Geometry: final body of the model. Coordinates: model frame, mm. Face numbers are marked on the shaded views. A direction names the side the tool comes from. Round coordinates to 2 decimals unless told otherwise and drop trailing zeros. Order: outer loops, then holes, each group sorted by start corner. A loop starts at its lowest first (then second) coordinate and runs counter-clockwise, first axis right, second up. Notation, with made-up numbers: (9.5, -6.75) - (29.5, -6.75) arc R9 ccw to (29.5, 7.25) - close; hole circle Ø1 at (-16.75, 37.25). An arc over 180 degrees is marked (long way). Put each result on its own line as item: value. Start each with the question number.
(1) Access query for the marked faces 1 and 2. Directions: +Z, -Z, +X, -X, +Y, -Y. A direction counts if a zero-diameter tool reaches every point of the face in a straight line with its end or side. Return the directions, or none.
(2) Pin query (flat end, axial travel): P1, Ø6, axis at x = 8, z = 40, coming from the +Y side; P2, Ø5, axis at y = 11.75, z = 9.5, coming from the -X side; P3, Ø10.5, axis at x = 45, y = 5.5, coming from the -Z side. Return the tip coordinate at first contact, or that it passes through.
(3) Material intervals for L1, parallel to Y at x = 51.85, z = 40.5; L2, parallel to Z at x = 51, y = 11; L3, parallel to Z at x = 54.05, y = 11.75, sorted ascending. Write a range as [from, to].
(4) Section C-C (x = 33). Output: boundary loops of the cut face in (y, z), and give its area (3 significant figures).
(5) Section D-D (y = 11). Output: boundary loops of the cut face in (x, z).
(6) Section A-A (z = 25). Output: boundary loops of the cut face in (x, y), and give its area (3 significant figures).
(7) Section B-B (y = 27.25). Output: boundary loops of the cut face in (x, z), and give its area (4 significant figures).
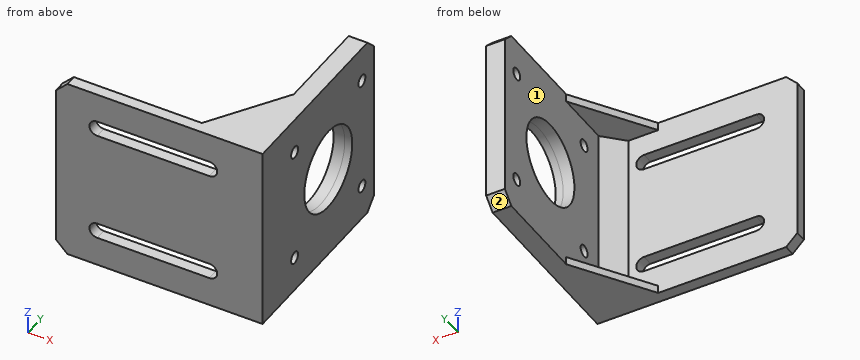
from build123d import *

# Parameters (mm, degrees)
EXTRUDE_1_DEPTH             = 50
HOLE_WIZARD_1_D             = 22.1
HOLE_WIZARD_1_DEPTH         = 100
HOLE_WIZARD_2_D             = 3.2
HOLE_WIZARD_2_DEPTH         = 100
HOLE_START                  = -3
HOLE_WIZARD_4_2_4_2_1_DEPTH = 3
RIB_1_REACH                 = 89.542
SKETCH_13_WALL_W            = 200.93798631
SKETCH_13_WALL_H            = 2.1
CHAMFER_1_SIZE              = 3
EXTRUDE_START               = 2
SKETCH_14_R                 = 1.6
SKETCH_14_R_2               = 11.05
EXTRUDE_2_DEPTH             = 2
CHAMFER_2_SIZE              = 5


# Read off the part's stored shape, not the designer's step: Ø4.2 (4.2) 直径槽口1
with BuildPart() as part:
    # 草图1 → 凸台-拉伸1 (new body)
    with BuildSketch(Plane.XY):
        Polygon((0, 0), (50.25, 0), (50.25, 48.25), (53.25, 48.25), (53.25, -3), (0, -3), align=None)
    extrude(amount=EXTRUDE_1_DEPTH)

    # 孔1
    with Locations(Plane.ZY.offset(-50.25)):
        with Locations((25, 27.25)):
            Hole(HOLE_WIZARD_1_D / 2, depth=HOLE_WIZARD_1_DEPTH)

    # 孔2
    with Locations(Plane.ZY.offset(-50.25)):
        with Locations((9.5, 42.75), (40.5, 42.75), (40.5, 11.75), (9.5, 11.75)):
            Hole(HOLE_WIZARD_2_D / 2, depth=HOLE_WIZARD_2_DEPTH)

    # Ø4.2 (4.2) 直径槽口1 outline → Ø4.2 (4.2) 直径槽口1 (cut)
    with BuildSketch(Plane(origin=(0, 0, 0), x_dir=(1, 0, 0), z_dir=(0, 1, 0)).offset(HOLE_START)):
        with BuildLine():
            Line((11, -42.1), (41, -42.1))
            ThreePointArc((41, -42.1), (43.1, -40), (41, -37.9))
            Line((41, -37.9), (11, -37.9))
            ThreePointArc((11, -37.9), (8.9, -40), (11, -42.1))
        make_face()
        with BuildLine():
            Line((11, -12.1), (41, -12.1))
            ThreePointArc((41, -12.1), (43.1, -10), (41, -7.9))
            Line((41, -7.9), (11, -7.9))
            ThreePointArc((11, -7.9), (8.9, -10), (11, -12.1))
        make_face()
    extrude(amount=HOLE_WIZARD_4_2_4_2_1_DEPTH, mode=Mode.SUBTRACT)

    # 草图13 wall → 筋1 (add, up to next)
    with BuildSketch(Plane(origin=(43.75, 10, 50), x_dir=(-0.544988350595, -0.838443616301, 0), z_dir=(0.838443616301, -0.544988350595, 0)), mode=Mode.PRIVATE) as rib_1_sk1:
        with Locations((0, 1.05)):
            Rectangle(SKETCH_13_WALL_W, SKETCH_13_WALL_H)
    rib_1_tool1 = extrude(rib_1_sk1.sketch, amount=RIB_1_REACH, mode=Mode.PRIVATE) - part.part
    rib_1 = rib_1_tool1.solids().sort_by_distance((43.75, 10, 50))[0]
    add(rib_1)

    # 镜向1: 筋1 across plane
    add(rib_1.mirror(Plane.XY.offset(25)))

    # 倒角1
    chamfer_1_edges = [part.edges().sort_by_distance(p)[0] for p in [
        (51.75, 48.25, 50),
        (0, -1.5, 50),
        (51.75, 48.25, 0),
        (0, -1.5, 0),
    ]]
    chamfer(chamfer_1_edges, length=CHAMFER_1_SIZE)

    # 草图14 → 凸台-拉伸2 (add)
    with BuildSketch(Plane(origin=(53.25, 0, 0), x_dir=(0, 0, -1), z_dir=(1, 0, 0)).offset(EXTRUDE_START)):
        Polygon((-47, 48.25), (-3, 48.25), (0, 45.25), (0, -3), (-50, -3), (-50, 45.25), align=None)
        with Locations(Location((-9.5, 42.75, 0), (0, 0, 180))):
            Circle(SKETCH_14_R, mode=Mode.SUBTRACT)
        with Locations(Location((-40.5, 42.75, 0), (0, 0, 180))):
            Circle(SKETCH_14_R, mode=Mode.SUBTRACT)
        with Locations(Location((-25, 27.25, 0), (0, 0, 180))):
            Circle(SKETCH_14_R_2, mode=Mode.SUBTRACT)
        with Locations(Location((-9.5, 11.75, 0), (0, 0, 180))):
            Circle(SKETCH_14_R, mode=Mode.SUBTRACT)
        with Locations(Location((-40.5, 11.75, 0), (0, 0, 180))):
            Circle(SKETCH_14_R, mode=Mode.SUBTRACT)
    extrude(amount=-EXTRUDE_2_DEPTH)

    # 倒角2
    chamfer_2_edges = [part.edges().sort_by_distance(p)[0] for p in [
        (50.25, 0, 25),
    ]]
    chamfer(chamfer_2_edges, length=CHAMFER_2_SIZE)


solid = part.part
Checks:
1. face 1: -X, +Y
1. face 2: -Z, +X, -X, +Y
2. P1: stops at y = 0
2. P2: stops at x = 50.25
2. P3: stops at z = 0
3. L1: y = [-3, 10.15], [13.35, 41.15], [44.35, 48.25]
3. L2: z = [0, 8.09], [10.91, 39.09], [41.91, 50]
3. L3: z = [0, 7.9], [11.1, 38.9], [42.1, 50]
4. outline: (-3, 0) - (0, 0) - (0, 7.9) - (-3, 7.9) - close; (-3, 12.1) - (0, 12.1) - (0, 37.9) - (-3, 37.9) - close; (-3, 42.1) - (0, 42.1) - (0, 50) - (-3, 50) - close
4. area: 125 mm²
5. outline: (44.4, 0) - (55.25, 0) - (55.25, 8.09) - (50.25, 8.09) - (50.25, 2.1) - (44.4, 2.1) - close; (44.4, 47.9) - (50.25, 47.9) - (50.25, 41.91) - (55.25, 41.91) - (55.25, 50) - (44.4, 50) - close; (50.25, 10.91) - (55.25, 10.91) - (55.25, 39.09) - (50.25, 39.09) - close
6. outline: (0, -3) - (55.25, -3) - (55.25, 16.2) - (50.25, 16.2) - (50.25, 5) - (45.25, 0) - (0, 0) - close; (50.25, 38.3) - (55.25, 38.3) - (55.25, 48.25) - (50.25, 48.25) - close
6. area: 309 mm²
7. outline: (50.25, 0) - (55.25, 0) - (55.25, 13.95) - (50.25, 13.95) - close; (50.25, 36.05) - (55.25, 36.05) - (55.25, 50) - (50.25, 50) - close
7. area: 139.5 mm²
